```python
from build123d import *

# Parameters (mm, degrees)
SKETCH1_R           = 57.15
SKETCH1_R_2         = 30.099
EXTRUDE_THIN1_DEPTH = 17.526
SKETCH2_R           = 4.2164
CUT_EXTRUDE2_DEPTH  = 17.526
CIRPATTERN1_COUNT   = 8


with BuildPart() as part:
    # Sketch1 → Extrude-Thin1 (new body)
    with BuildSketch(Plane(origin=(0, 0, 0), x_dir=(1, 0, 0), z_dir=(0, 1, 0))):
        Circle(SKETCH1_R)
        Circle(SKETCH1_R_2, mode=Mode.SUBTRACT)
    extrude(amount=EXTRUDE_THIN1_DEPTH)

    # Sketch2 → Cut-Extrude2 (cut)
    with BuildSketch(Plane(origin=(0, 0, 0), x_dir=(1, 0, 0), z_dir=(0, 1, 0))):
        with Locations((0, 46.101)):
            Circle(SKETCH2_R)
    cut_extrude2 = extrude(amount=CUT_EXTRUDE2_DEPTH, mode=Mode.SUBTRACT)

    # CirPattern1: Cut-Extrude2 ×8 about axis
    cirpattern1_axis = Axis((0, 0, 0), (0, 1, 0))
    for i in range(1, CIRPATTERN1_COUNT):
        add(cut_extrude2.rotate(cirpattern1_axis, i * 360 / CIRPATTERN1_COUNT), mode=Mode.SUBTRACT)


solid = part.part
```
For this review, take the finished solid that the model builds, in its own axes (mm). Round coordinates to 2 decimals unless told otherwise and drop trailing zeros. Write each loop counter-clockwise with the first axis right and the second up, starting at its lowest first coordinate (ties: lowest second). Pieces come first, ordered by that corner, then holes. Notation, with made-up numbers: (-26.5, 34) -> (-7.5, 34) arc R20 cw to (-7.5, 67) -> close; hole circle Ø6 at (31.25, -34.5). An arc over 180 degrees is marked (long way). Use one line per item in the form item = value.
1) Take a section at A-A, the plane z = 0. Write out the cut boundary in (x, y), and give its area (3 significant figures).
Found:
outline = (-57.15, 0) -> (-50.32, 0) -> (-50.32, 17.53) -> (-57.15, 17.53) -> close; (-41.88, 0) -> (-30.1, 0) -> (-30.1, 17.53) -> (-41.88, 17.53) -> close; (30.1, 0) -> (41.88, 0) -> (41.88, 17.53) -> (30.1, 17.53) -> close; (50.32, 0) -> (57.15, 0) -> (57.15, 17.53) -> (50.32, 17.53) -> close
area = 653 mm2
2) Clearance check with flat-ended pins moving along their axes: pin 1 (3 mm diameter, centred on x = 28, y = 16, fed in from +Z); pin 2 (10 mm diameter, centred on y = 3, z = 41.5, fed in from -X); pin 3 (10 mm diameter, centred on x = -36.5, y = 3.5, fed in from -Z); pin 4 (3 mm diameter, centred on y = 3, z = 1.5, fed in from +X). State where each tip first meets the part, or that it passes through.
Found:
pin_1 = 50.63
pin_2 = -43.98
pin_3 = -47.69
pin_4 = 57.15
3) Mouldability with a two-part tool opening along X and no side actions: class faces 1 (the cylindrical face through (-57.095, 8.64, -2.513)), 2 (the flat face through (25, 0, 25)), 3 (the cylindrical face through (32.42, 8.64, -36.81)) as +X half, -X half, draft (parallel to the pull), parting line (faces both ways), or undercut.
Found:
face_1 = parting line
face_2 = draft
face_3 = undercut
4) Take a section at B-B, the plane x = 0. Write out the cut boundary in (y, z), and give its area (3 significant figures).
Found:
outline = (0, -57.15) -> (17.53, -57.15) -> (17.53, -50.32) -> (0, -50.32) -> close; (0, -41.88) -> (17.53, -41.88) -> (17.53, -30.1) -> (0, -30.1) -> close; (0, 30.1) -> (17.53, 30.1) -> (17.53, 41.88) -> (0, 41.88) -> close; (0, 50.32) -> (17.53, 50.32) -> (17.53, 57.15) -> (0, 57.15) -> close
area = 653 mm2
5) Take a section at C-C, the plane x = -22. Write out the cut boundary in (y, z), and give its area (3 significant figures).
Found:
outline = (0, -52.75) -> (17.53, -52.75) -> (17.53, -20.54) -> (0, -20.54) -> close; (0, 20.54) -> (17.53, 20.54) -> (17.53, 52.75) -> (0, 52.75) -> close
area = 1,130 mm2
6) To check wall thickness, follow L1, parallel to X at y = 11.5, z = 0; L2, parallel to Z at x = 13, y = 13. State the ranges of each line that lie inside material, in increasing order. Write a range as from..to.
Found:
L1 = -57.15..-50.32, -41.88..-30.1, 30.1..41.88, 50.32..57.15
L2 = -55.65..-27.15, 27.15..55.65
7) Take a section at D-D, the plane y = 15.75. Count the separate pieces of the cut face and the enclosed holes in it, and give its area (3 significant figures).
Found:
separate_pieces = 1
enclosed_holes = 9
area = 6,970 mm2
